Can you work these out from the model? Positions are in its coordinate system, mm. Face numbers are marked on the shaded views. A direction names the side the tool comes from. Give positions to 0.01 mm unless a question says otherwise; leave off trailing zeros. Order: outer loops, then holes, each group sorted by start corner. A loop starts at its lowest first (then second) coordinate and runs counter-clockwise, first axis right, second up. Notation, with made-up numbers: M 70,43.5 L 81,43.5 A15 cw 81,72.5 Z; hole C -8,0.25 d8. An arc over 180 degrees is marked long. Answer as a JSON object with one key per item and string values.
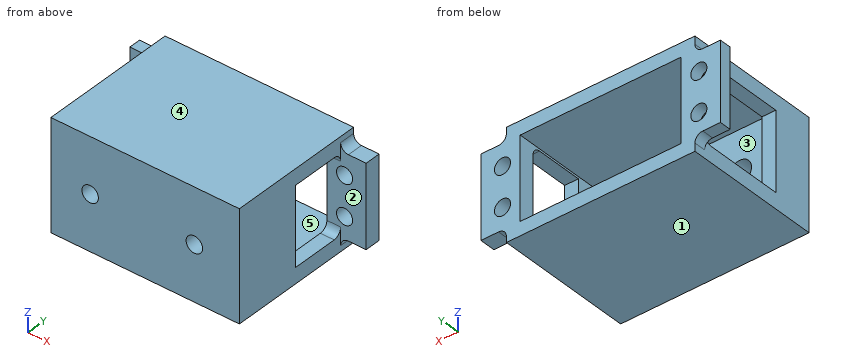
```python
from build123d import *

# Parameters (mm, degrees)
SKETCH_1_W               = 48
SKETCH_1_H               = 28
EXTRUDE_1_DEPTH          = 9.3
SKETCH_2_W               = 48
SKETCH_2_H               = 28
SKETCH_2_W_2             = 40
SKETCH_2_H_2             = 20
EXTRUDE_2_DEPTH          = 26
SKETCH_3_W               = 41
SKETCH_3_H               = 21
CUT_EXTRUDE_1_DEPTH      = 26
SKETCH_4_W               = 19.956885432
SKETCH_4_H               = 18
CUT_EXTRUDE_2_DEPTH      = 10
CUT_EXTRUDE_3_DEPTH      = 6
SKETCH_7_W               = 20
SKETCH_7_H               = 3
EXTRUDE_4_DEPTH          = 10
FILLET_3_R               = 2
SKETCH_9_W               = 21
SKETCH_9_H               = 4
EXTRUDE_5_DEPTH          = 10
SKETCH_10_R              = 2.05
CUT_EXTRUDE_5_DEPTH      = 10
FILLET_4_R               = 2
SKETCH_11_R              = 3
CUT_EXTRUDE_6_DEPTH      = 5.3
CUT_EXTRUDE_7_DEPTH      = 46.890521897
CUT_EXTRUDE_7_DEPTH_BACK = 46.890521897
SKETCH_12_R              = 2.1
FILLET_5_R               = 2


with BuildPart() as part:
    # 草图1 → 凸台-拉伸1 (new body)
    with BuildSketch(Plane(origin=(0, 0, 0), x_dir=(1, 0, 0), z_dir=(0, 1, 0))):
        Rectangle(SKETCH_1_W, SKETCH_1_H)
    extrude(amount=EXTRUDE_1_DEPTH)

    # 草图2 → 凸台-拉伸2 (add)
    with BuildSketch(Plane(origin=(0, 9.3, 0), x_dir=(1, 0, 0), z_dir=(0, 1, 0))):
        Rectangle(SKETCH_2_W, SKETCH_2_H)
        Rectangle(SKETCH_2_W_2, SKETCH_2_H_2, mode=Mode.SUBTRACT)
    extrude(amount=EXTRUDE_2_DEPTH)

    # 草图3 → 切除-拉伸1 (cut)
    with BuildSketch(Plane(origin=(0, 35.3, 0), x_dir=(1, 0, 0), z_dir=(0, 1, 0))):
        Rectangle(SKETCH_3_W, SKETCH_3_H)
    extrude(amount=-CUT_EXTRUDE_1_DEPTH, mode=Mode.SUBTRACT)

    # 草图4 → 切除-拉伸2 (cut)
    with BuildSketch(Plane(origin=(24, 0, 0), x_dir=(0, 0, -1), z_dir=(1, 0, 0))):
        with Locations((0.021557284, 26.3)):
            Rectangle(SKETCH_4_W, SKETCH_4_H)
    extrude(amount=-CUT_EXTRUDE_2_DEPTH, mode=Mode.SUBTRACT)

    # 草图6 → 切除-拉伸3 (cut)
    with BuildSketch(Plane.ZY.offset(24)):
        Polygon((0, 35.3), (-10, 35.3), (-10, 10.3), (10, 10.3), (10, 35.3), align=None)
    extrude(amount=-CUT_EXTRUDE_3_DEPTH, mode=Mode.SUBTRACT)

    # 草图7 → 凸台-拉伸4 (add)
    with BuildSketch(Plane(origin=(-20.5, 0, 0), x_dir=(0, 0, -1), z_dir=(1, 0, 0))):
        with Locations((0, 33.8)):
            Rectangle(SKETCH_7_W, SKETCH_7_H)
    extrude(amount=-EXTRUDE_4_DEPTH)

    # 圆角3
    fillet_3_edges = [part.edges().sort_by_distance(p)[0] for p in [
        (-24, 33.8, 10),
        (-24, 33.8, -10),
    ]]
    fillet(fillet_3_edges, radius=FILLET_3_R)

    # 草图9 → 凸台-拉伸5 (add)
    with BuildSketch(Plane.ZY.offset(-20.5)):
        with Locations((0, 33.3)):
            Rectangle(SKETCH_9_W, SKETCH_9_H)
    extrude(amount=-EXTRUDE_5_DEPTH)

    # 草图10 → 切除-拉伸5 (cut)
    with BuildSketch(Plane(origin=(0, 35.3, 0), x_dir=(1, 0, 0), z_dir=(0, 1, 0))):
        with Locations(Location((25, 5, 0), (0, 0, 270))):
            Circle(SKETCH_10_R)
        with Locations(Location((25, -5, 0), (0, 0, 270))):
            Circle(SKETCH_10_R)
        with Locations(Location((-25, 5, 0), (0, 0, 270))):
            Circle(SKETCH_10_R)
        with Locations(Location((-25, -5, 0), (0, 0, 270))):
            Circle(SKETCH_10_R)
    extrude(amount=-CUT_EXTRUDE_5_DEPTH, mode=Mode.SUBTRACT)

    # 圆角4
    fillet_4_edges = [part.edges().sort_by_distance(p)[0] for p in [
        (24, 33.3, -10.5),
        (24, 33.3, 10.5),
    ]]
    fillet(fillet_4_edges, radius=FILLET_4_R)

    # 草图11 → 切除-拉伸6 (cut)
    with BuildSketch(Plane(origin=(0, 9.3, 0), x_dir=(1, 0, 0), z_dir=(0, 1, 0))):
        with Locations(Location((-14, 0, 0), (0, 0, 270))):
            Circle(SKETCH_11_R)
        with Locations(Location((12.529194913, 0, 0), (0, 0, 270))):
            Circle(SKETCH_11_R)
    extrude(amount=-CUT_EXTRUDE_6_DEPTH, mode=Mode.SUBTRACT)

    # 草图12 → 切除-拉伸7 (cut, two sides: drawn at the far end of the back side and taken through both)
    with BuildSketch(Plane(origin=(0, 4, 0), x_dir=(1, 0, 0), z_dir=(0, 1, 0)).offset(-CUT_EXTRUDE_7_DEPTH_BACK)):
        with Locations(Location((-14, 0, 0), (0, 0, 270))):
            Circle(SKETCH_12_R)
        with Locations(Location((12.529194913, 0, 0), (0, 0, 270))):
            Circle(SKETCH_12_R)
    extrude(amount=CUT_EXTRUDE_7_DEPTH + CUT_EXTRUDE_7_DEPTH_BACK, mode=Mode.SUBTRACT)

    # 圆角5
    fillet_5_edges = [part.edges().sort_by_distance(p)[0] for p in [
        (-22.25, 32.3, -10),
        (-22.25, 32.3, 10),
        (22.25, 31.3, 9.956885432),
        (22.25, 31.3, -10),
    ]]
    fillet(fillet_5_edges, radius=FILLET_5_R)


solid = part.part
```
1) I want a section at C-C on z = 4.75. Write out the boundary of the cut face in (x, y), and give its area (3 significant figures).
Results found:
{"outline": "M -30.5,32.3 L -27.03,32.3 L -27.03,35.3 L -30.5,35.3 Z; M -24,0 L 24,0 L 24,17.3 L 20.5,17.3 L 20.5,9.3 L -20.5,9.3 L -20.5,10.3 L -24,10.3 Z; M -22.97,32.3 L -20.5,32.3 L -20.5,35.3 L -22.97,35.3 Z; M 20.5,31.3 L 22.97,31.3 L 22.97,35.3 L 20.5,35.3 Z; M 27.03,31.3 L 30.5,31.3 L 30.5,35.3 L 27.03,35.3 Z", "area": "519 mm²"}
2) Thinking about a two-plate mould opening in Y: for the marked faces 1, 2 and 3, which applies, pulls with the +Y half, pulls with the -Y half, needs draft (parallel to the pull), parting line crosses it, or undercut?
Results found:
{"face 1": "needs draft", "face 2": "undercut", "face 3": "pulls with the +Y half"}
3) For the marked faces 4 and 5, which set-ups out of +Z, -Z, +X, -X, +Y, -Y let a thin tool reach every point of the face, with its end or its side?
Results found:
{"face 4": "+Z, +X, -X, +Y, -Y", "face 5": "+Y"}
4) I need wall thicknesses on L1, parallel to X at y = 32.9, z = 5; L2, parallel to X at y = 1.95, z = 0; L3, parallel to X at y = 7.85, z = 0. Which ranges of each line are inside material? Lowest first, please.
Results found:
{"L1": "x = -30.5 to -27.05, -22.95 to -20.5, 20.5 to 22.95, 27.05 to 30.5", "L2": "x = -24 to -16.1, -11.9 to 10.43, 14.63 to 24", "L3": "x = -24 to -17, -11 to 9.53, 15.53 to 24"}
5) I want a section at B-B on y = 33.5. Write out the boundary of the cut face in (x, z), and give its area (3 significant figures).
Results found:
{"outline": "M -30.5,-10 L -26,-10 A2 cw -24,-12 L -24,-14 L 24,-14 L 24,-12.5 A2 cw 26,-10.5 L 30.5,-10.5 L 30.5,10.5 L 26,10.5 A2 cw 24,12.5 L 24,14 L -24,14 L -24,12 A2 cw -26,10 L -30.5,10 Z; hole C -25,-5 d4.1; hole C -25,5 d4.1; hole M -20.5,-10.5 L 20.5,-10.5 L 20.5,10.5 L -20.5,10.5 Z; hole C 25,-5 d4.1; hole C 25,5 d4.1", "area": "700 mm²"}
6) I'm going to push flat-ended pins straight in: pin 1 Ø1 at (y, z) = (29.5, 11) entering from -X; pin 2 Ø5 at (x, z) = (11.5, -0.5) entering from +Y; pin 3 Ø1 at (y, z) = (29.5, 9) entering from +X; pin 4 Ø2.5 at (x, z) = (-25, 5) entering from +Y. Where does each tip first touch, or does it pass through?
Results found:
{"pin 1": "stops at x = -24", "pin 2": "stops at y = 9.3", "pin 3": "passes through", "pin 4": "stops at y = 10.3"}
7) I want a section at A-A on x = -14. Write out the boundary of the cut face in (y, z).
Results found:
{"outline": "M 0,-14 L 35.3,-14 L 35.3,-10.5 L 9.3,-10.5 L 9.3,-3 L 4,-3 L 4,-2.1 L 0,-2.1 Z; M 0,2.1 L 4,2.1 L 4,3 L 9.3,3 L 9.3,10.5 L 35.3,10.5 L 35.3,14 L 0,14 Z"}
8) I want a section at D-D on x = 25. Write out the boundary of the cut face in (y, z).
Results found:
{"outline": "M 31.3,-10.77 L 35.3,-10.77 L 35.3,-7.05 L 31.3,-7.05 Z; M 31.3,-2.95 L 35.3,-2.95 L 35.3,2.95 L 31.3,2.95 Z; M 31.3,7.05 L 35.3,7.05 L 35.3,10.77 L 31.3,10.77 Z"}
